Could you check a few things on this model? Use its own coordinates, in mm. Face numbers are marked on the shaded views. A direction names the side the tool comes from. Coordinates: 2 decimals unless noted, no trailing zeros. Write each loop counter-clockwise with the first axis right and the second up, starting at its lowest first coordinate (ties: lowest second). Pieces come first, ordered by that corner, then holes.
Item 1: Which directions (+Z, -Z, +X, -X, +Y, -Y) give clear straight access to the entire face, cutting with the end or side of a thin tool? Please do the marked faces 1, 2 and 3.
Item 2: For P1, Ø3, axis at x = 84.5, y = -18, coming from the +Z side; P2, Ø12, axis at y = 11.5, z = 52, coming from the +X side; P3, Ø12, axis at x = 18.5, y = -30, coming from the -Z side; P4, Ø1, axis at y = 9, z = 52, coming from the +X side, each with a flat end and sliding along its axis, tell me the tip position at first contact or that it passes through.
Item 3: I want a section at C-C on y = -12. Please give me the cut outline in (x, z), then the cut area to 3 significant figures.
Item 4: I want a section at B-B on x = 8. Please give me the cut outline in (y, z).
Item 5: I want a section at A-A on z = 7. Please give me the cut outline in (x, y) (3 decimals).
Item 6: If I drill on probe 1 along Y at (x, z) = (54.5, 65.5); probe 2 along X at (y, z) = (-11.5, 37.5); probe 3 along Z at (x, y) = (88.5, 3.5), over which ranges is the centre line in solid material (lowest first)?
Item 7: I want a section at D-D on z = 34. Please give me the cut outline in (x, y).
from build123d import *

# Parameters (mm, degrees)
SKETCH1_W      = 30
SKETCH1_H      = 40
SKETCH1_W_2    = 50
REVOLVE8_ANGLE = 90


with BuildPart() as part:
    # Sketch1 → Revolve8 (revolve)
    with BuildSketch(Plane.XY):
        Polygon((40, 34.160621762), (0, 34.160621762), (0, -41.839378238), (20, -41.839378238), (20, -31.839378238), (20, 29.160621762), (40, 29.160621762), align=None)
        Polygon((40, 28.160621762), (40, 29.160621762), (20, 29.160621762), (20, -31.839378238), (21, -31.839378238), (21, -21.839378238), (21, 18.160621762), (21, 28.160621762), align=None)
        Polygon((101, 28.160621762), (40, 28.160621762), (21, 28.160621762), (21, 18.160621762), (51, 18.160621762), (101, 18.160621762), align=None)
        Polygon((21, -21.839378238), (21, -31.839378238), (101, -31.839378238), (101, -21.839378238), (51, -21.839378238), align=None)
        with Locations((36, -1.839378238)):
            Rectangle(SKETCH1_W, SKETCH1_H)
        with Locations((76, -1.839378238)):
            Rectangle(SKETCH1_W_2, SKETCH1_H)
    revolve(axis=Axis((0, 34.160621762, 0), (0, -1, 0)), revolution_arc=REVOLVE8_ANGLE)


solid = part.part
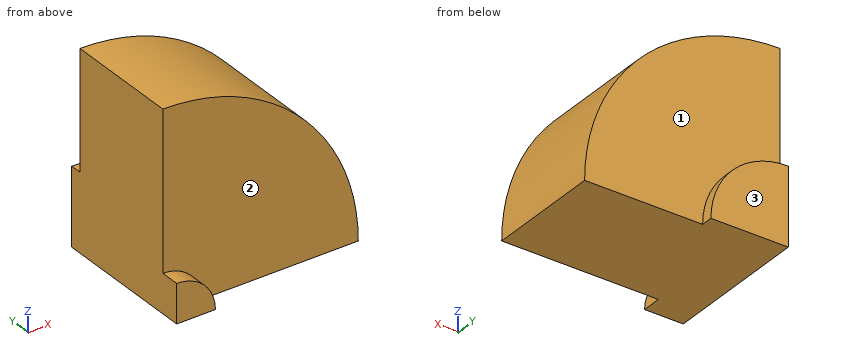
Response values:
1. face 1: +Z, +X, +Y
1. face 2: +Z, +X, -Y
1. face 3: +Z, -Z, +X, -X, +Y
2. P1: stops at z = 57.55
2. P2: stops at x = 89.92
2. P3: stops at z = 0
2. P4: stops at x = 86.88
3. outline: (0, 0) - (101, 0) arc R101 ccw to (0, 101) - close
3. area: 8,010 mm2
4. outline: (-41.84, 0) - (34.16, 0) - (34.16, 39.19) - (28.16, 39.19) - (28.16, 100.68) - (-31.84, 100.68) - (-31.84, 18.33) - (-41.84, 18.33) - close
5. outline: (0, -41.839) - (18.735, -41.839) - (18.735, -31.839) - (100.757, -31.839) - (100.757, 28.161) - (39.383, 28.161) - (39.383, 34.161) - (0, 34.161) - close
6. probe 1: y = -31.84 to 28.16
6. probe 2: x = 0 to 93.78
6. probe 3: z = 0 to 48.67
7. outline: (0, -31.84) - (95.11, -31.84) - (95.11, 28.16) - (21.07, 28.16) - (21.07, 34.16) - (0, 34.16) - close
